Source: CAD feature listing. Evaluate the final solid. Frame: model axes, mm. A direction names the side the tool comes from. Round coordinates to 2 decimals unless told otherwise and drop trailing zeros. Loops run counter-clockwise (first coordinate to the right, second up) from the corner with the lowest first, then second, coordinate; pieces in that order, holes last. Notation, with made-up numbers: (-22.75, 42) -> (27.25, 42) arc R13 ccw to (27.25, 49) -> close; hole circle Ø9 at (32.5, 67.25). An arc over 180 degrees is marked (long way). Put each result on its own line as item: value. Start each with the question number.
1. Material intervals for L1, parallel to X at y = 10, z = 6.5 (3 decimals); L2, parallel to Y at x = 15, z = 3.5 (3 decimals); L3, parallel to X at y = 47, z = 7, sorted ascending.
2. Cut plane C-C (z = 37). Return the cut outline in (x, y).
3. Contact query for flat-ended pins moving along their axis: pin 1 (6 mm diameter, centred on y = -9.5, z = 6, fed in from +X); pin 2 (10 mm diameter, centred on x = 15, y = 10, fed in from +Z); pin 3 (12 mm diameter, centred on x = 10, y = 29.5, fed in from +Z). Output: stop coordinate, or through.
4. Cut plane D-D (y = 67.5). Return the cut outline in (x, z), then the cut area to 3 significant figures.
5. Set-up query: faces 1 (the flat face through (30, -10, 4)), 2 (the flat face through (18, -1, 8)), 3 (the flat face through (0, 39, 15)). Return all of +Z, -Z, +X, -X, +Y, -Y with unobstructed straight access to the full face (end or side cutting, diameter ignored); none if empty.
6. Cut plane B-B (x = 15). State how many separate pieces and enclosed holes the cut face has, then the cut area to 3 significant figures.
7. Draft query along Y for faces 4 (the cylindrical face through (12.52, -3.1, 3.94)), 5 (the flat face through (37, 42, 40)), 6 (the flat face through (15, -19.278, 4)), 7 (the cylindrical face through (12.52, 11.9, 3.94)). Return one class per face: pulls with the +Y half, pulls with the -Y half, needs draft (parallel to the pull), parting line crosses it, or undercut.
8. Cut plane A-A (y = -5). Return the cut outline in (x, z) (3 decimals), then the cut area to 3 significant figures.
Autodesk Inventor part; units mm, degrees
ref_plane "YZ Plane" through (0, 0, 0) normal (1, 0, 0) x (0, 1, 0)
ref_plane "XZ Plane" through (0, 0, 0) normal (0, 1, 0) x (-1, 0, 0)
ref_plane "XY Plane" through (0, 0, 0) normal (0, 0, 1) x (1, 0, 0)
sketch "Sketch1" plane through (0, 0, 0) normal (0, 0, 1) x (1, 0, 0)
  line L0 (0, 0) -> (30, 0)
  line L1 (30, 0) -> (30, 40)
  line L2 (30, 40) -> (0, 40)
  line L3 (0, 40) -> (0, 0)
  circle A0 centre (15, 10) radius 3.125
  circle A1 centre (15, -5) radius 3.125
  line L4 (51.875, 74) -> (51.875, 6) construction
  line L5 (51.875, 6) -> (16.525, 6) construction
  line L6 (16.525, 6) -> (16.525, 74)
  line L7 (51.875, 40) -> (34.2, 40)
  line L8 (34.2, 40) -> (34.2, 75.5)
  circle A2 centre (34.2, 75.5) radius 32.5
  line L9 (0, 40) -> (68.4124, 40)
  line L10 (68.4124, 40) -> (68.4124, 75.5)
  line L11 (68.4124, 75.5) -> (0, 75.5)
  line L12 (0, 75.5) -> (0, 40)
  line L13 (68.4124, 40) -> (30, 0)
  line L14 (0, 40) -> (30, 40)
  line L15 (30, 40) -> (30, -19.2784)
  line L16 (30, -19.2784) -> (0, -19.2784)
  line L17 (0, -19.2784) -> (0, 40)
  point P0 (15, 40)
  point P1 (34.2062, 75.5)
  point P2 (1.7, 75.5)
  point P3 (66.7, 75.5)
  dimension "d0" = 30
  dimension "d1" = 15
  dimension "d2" = 15
  dimension "d3" = 40
  dimension "d4" = 6.25
  dimension "d5" = 6.25
  dimension "d6" = 30
  dimension "d7" = 35.35
  dimension "d8" = 13.475
  dimension "d10" = 34
  dimension "d11" = 35.5
  dimension "d12" = 65
  dimension "d13" = 34.2062
  dimension "d15" = 34.2062
extrude "Extrusion1" add sketch "Sketch1" along normal blind 8 contours L3 L2 L1 L0 | L0 L15 L16 L17 | L1 L9 L7 L13 | L12 L11 A2 L6 L2 | L2 L6 A2 L8 L9 | L9 L7 L8 A2 L11 L10
extrude "Extrusion2" add sketch "Sketch1" along normal blind 40 contours L12 L11 A2 L6 L2 | L2 L6 A2 L8 L9 | L9 L7 L8 A2 L11 L10
chamfer "Chamfer1" distance 32 angle 35 1 edges at (34.2062, 40, 8) measured on face at (22.8041, 40, 18.6667)
properties part number "motorsupport"
Solution:
1. L1: x = 0 to 11.875, 18.125 to 39.603
1. L2: y = -19.278 to -8.125, -1.875 to 6.875, 13.125 to 49.278
1. L3: x = 0 to 18.58, 49.82 to 68.41
2. outline: (0, 37.9) -> (66.4, 37.9) -> (68.41, 40) -> (68.41, 75.5) -> (66.7, 75.5) arc R32.5 cw to (1.7, 75.5) -> (0, 75.5) -> close
3. pin 1: stops at x = 30
3. pin 2: stops at z = 8
3. pin 3: stops at z = 33.57
4. outline: (0, 0) -> (2.7, 0) -> (2.7, 40) -> (0, 40) -> close; (65.7, 0) -> (68.41, 0) -> (68.41, 40) -> (65.7, 40) -> close
4. area: 216 mm^2
5. face 1: +Z, -Z, +X, -Y
5. face 2: +Z, +X, -X, -Y
5. face 3: +Z, -Z, -X, +Y, -Y
6. separate pieces: 3
6. enclosed holes: 0
6. area: 1,100 mm^2
7. face 4: undercut
7. face 5: needs draft
7. face 6: pulls with the -Y half
7. face 7: undercut
8. outline: (0, 0) -> (11.875, 0) -> (11.875, 8) -> (0, 8) -> close; (18.125, 0) -> (30, 0) -> (30, 8) -> (18.125, 8) -> close
8. area: 190 mm^2
